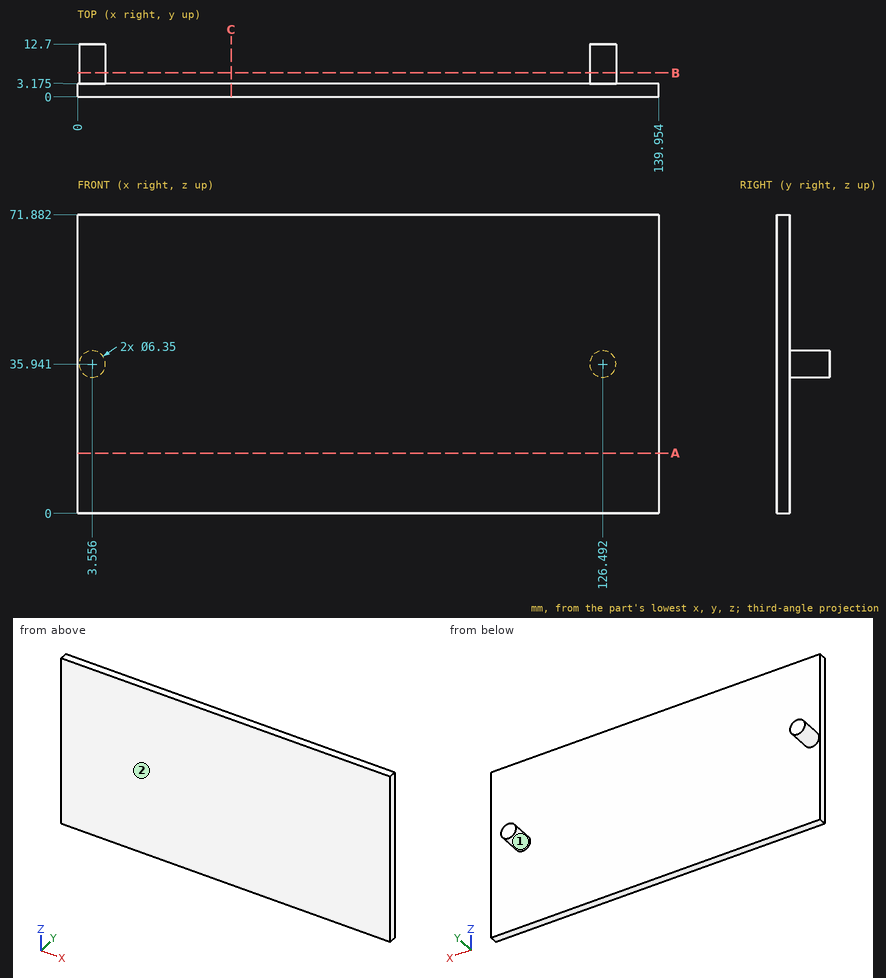
The drawing under review shows one solid part. Ordinate dimensions are in mm from its lowest x, y, z. Round coordinates to 2 decimals unless told otherwise and drop trailing zeros. Loops run counter-clockwise (first coordinate to the right, second up) from the corner with the lowest first, then second, coordinate; pieces in that order, holes last. Notation, with made-up numbers: (46, 53) - (71, 53) arc R23 cw to (71, 70) - close; hole circle Ø8 at (66, 37). An arc over 180 degrees is marked (long way). Put each result on its own line as item: value. Start each with the question number.
1. Consider section B-B on y = 5.75. State the section outline as (x, z) points (3 decimals), plus the area to 3 significant figures.
2. Consider section C-C on x = 37. State the section outline as (y, z) points (3 decimals).
3. Consider section A-A on z = 14.5. State the section outline as (x, y) points (3 decimals), plus the area to 3 significant figures.
4. Mouldability with a two-part tool opening along X and no side actions: class the marked faces 1 and 2 as +X half, -X half, draft (parallel to the pull), parting line (faces both ways), or undercut.
5. For probe 1 along Y at (x, z) = (109, 51.5) (3 decimals), list the stretches that pass through material, from the lowest coordinate up. Write a range as [from, to].
Result sheet:
1. outline: circle Ø6.35 at (3.556, 35.941); circle Ø6.35 at (126.492, 35.941)
1. area: 63.3 mm^2
2. outline: (0, 0) - (3.175, 0) - (3.175, 71.882) - (0, 71.882) - close
3. outline: (0, 0) - (139.954, 0) - (139.954, 3.175) - (0, 3.175) - close
3. area: 444 mm^2
4. face 1: undercut
4. face 2: draft
5. probe 1: [0, 3.175]
